Geometry check sheet. Reference: the model listing, model coordinates, mm. A direction names the side the tool comes from. Round coordinates to 2 decimals unless told otherwise and drop trailing zeros. Write each loop counter-clockwise with the first axis right and the second up, starting at its lowest first coordinate (ties: lowest second). Pieces come first, ordered by that corner, then holes. Notation, with made-up numbers: (46, -2.75) -> (70, -2.75) arc R11 ccw to (70, 2.25) -> close; hole circle Ø10 at (50.25, -6.75). An arc over 180 degrees is marked (long way). One line per question, with ' | ' between items.
```python
from build123d import *

# Parameters (mm, degrees)
SKETCH1_W                 = 50.8
SKETCH1_H                 = 126.238
BACK_DEPTH                = 3.175
CUT_EXTRUDE3_DEPTH        = 69.11203114
F_4_CLEARANCE_HOLE1_D     = 3.4544
LPATTERN1_OUTLINE_R       = 1.7272
LPATTERN1_DEPTH           = 3.175
SKETCH9_W                 = 55.88
SKETCH9_H                 = 131.318
WALLS_DEPTH               = 11.405821857
SKETCH11_W                = 69.85
SKETCH11_H                = 137.668
SKETCH11_W_2              = 50.8
SKETCH11_H_2              = 126.238
LIP_DEPTH                 = 2.54
F_6_CLEARANCE_OVERSIZED_D = 4.3053
FILLET2_R                 = 1.5875
CUT_EXTRUDE4_DEPTH        = 6.858
CUT_EXTRUDE4_DEPTH_BACK   = 3.81
SKETCH19_W                = 76.814856898
SKETCH19_H                = 21.095936882


# Read off the part's stored shape, not the designer's step: LPattern1
with BuildPart() as part:
    # Sketch1 → back (new body)
    with BuildSketch(Plane.XY):
        Rectangle(SKETCH1_W, SKETCH1_H)
    extrude(amount=BACK_DEPTH)

    # Sketch6 → Cut-Extrude3 (cut, through all)
    with BuildSketch(Plane.XY.offset(3.175)):
        with BuildLine():
            Line((24.07, -52.705), (24.07, 52.705))
            ThreePointArc((24.07, 52.705), (23.605032015, 53.827532015), (22.4825, 54.2925))
            Line((22.4825, 54.2925), (15.6245, 54.2925))
            ThreePointArc((15.6245, 54.2925), (14.501967985, 53.827532015), (14.037, 52.705))
            Line((14.037, 52.705), (14.037, -52.705))
            ThreePointArc((14.037, -52.705), (14.501967985, -53.827532015), (15.6245, -54.2925))
            Line((15.6245, -54.2925), (22.4825, -54.2925))
            ThreePointArc((22.4825, -54.2925), (23.605032015, -53.827532015), (24.07, -52.705))
        make_face()
    extrude(amount=-CUT_EXTRUDE3_DEPTH, mode=Mode.SUBTRACT)

    # #4 Clearance Hole1 (through all)
    with Locations(Plane(origin=(19.0535, 58.1025, 3.175), x_dir=(1, 0, 0), z_dir=(0, 0, 1))):
        with Locations((0, 0), (0, -116.205)):
            Hole(F_4_CLEARANCE_HOLE1_D / 2)

    # LPattern1 outline → LPattern1 (cut)
    with BuildSketch(Plane.XY):
        with BuildLine():
            ThreePointArc((1.337, -52.705), (1.801967985, -53.827532015), (2.9245, -54.2925))
            Line((2.9245, -54.2925), (9.7825, -54.2925))
            ThreePointArc((9.7825, -54.2925), (10.905032015, -53.827532015), (11.37, -52.705))
            Line((11.37, -52.705), (11.37, 52.705))
            ThreePointArc((11.37, 52.705), (10.905032015, 53.827532015), (9.7825, 54.2925))
            Line((9.7825, 54.2925), (2.9245, 54.2925))
            ThreePointArc((2.9245, 54.2925), (1.801967985, 53.827532015), (1.337, 52.705))
            Line((1.337, 52.705), (1.337, -52.705))
        make_face()
        with BuildLine():
            ThreePointArc((-11.363, -52.705), (-10.898032015, -53.827532015), (-9.7755, -54.2925))
            Line((-9.7755, -54.2925), (-2.9175, -54.2925))
            ThreePointArc((-2.9175, -54.2925), (-1.794967985, -53.827532015), (-1.33, -52.705))
            Line((-1.33, -52.705), (-1.33, 52.705))
            ThreePointArc((-1.33, 52.705), (-1.794967985, 53.827532015), (-2.9175, 54.2925))
            Line((-2.9175, 54.2925), (-9.7755, 54.2925))
            ThreePointArc((-9.7755, 54.2925), (-10.898032015, 53.827532015), (-11.363, 52.705))
            Line((-11.363, 52.705), (-11.363, -52.705))
        make_face()
        with BuildLine():
            ThreePointArc((-24.063, -52.705), (-23.598032015, -53.827532015), (-22.4755, -54.2925))
            Line((-22.4755, -54.2925), (-15.6175, -54.2925))
            ThreePointArc((-15.6175, -54.2925), (-14.494967985, -53.827532015), (-14.03, -52.705))
            Line((-14.03, -52.705), (-14.03, 52.705))
            ThreePointArc((-14.03, 52.705), (-14.494967985, 53.827532015), (-15.6175, 54.2925))
            Line((-15.6175, 54.2925), (-22.4755, 54.2925))
            ThreePointArc((-22.4755, 54.2925), (-23.598032015, 53.827532015), (-24.063, 52.705))
            Line((-24.063, 52.705), (-24.063, -52.705))
        make_face()
        with Locations((6.3535, -58.1025)):
            Circle(LPATTERN1_OUTLINE_R)
        with Locations((-6.3465, -58.1025)):
            Circle(LPATTERN1_OUTLINE_R)
        with Locations((-19.0465, -58.1025)):
            Circle(LPATTERN1_OUTLINE_R)
        with Locations((6.3535, 58.1025)):
            Circle(LPATTERN1_OUTLINE_R)
        with Locations((-6.3465, 58.1025)):
            Circle(LPATTERN1_OUTLINE_R)
        with Locations((-19.0465, 58.1025)):
            Circle(LPATTERN1_OUTLINE_R)
    extrude(amount=LPATTERN1_DEPTH, mode=Mode.SUBTRACT)

    # Sketch9 → walls (add)
    with BuildSketch(Plane.XY.offset(3.175)):
        Rectangle(SKETCH9_W, SKETCH9_H)
        with BuildLine():
            Line((25.4, -61.5315), (25.4, 61.5315))
            ThreePointArc((25.4, 61.5315), (24.935032015, 62.654032015), (23.8125, 63.119))
            Line((23.8125, 63.119), (-23.8125, 63.119))
            ThreePointArc((-23.8125, 63.119), (-24.935032015, 62.654032015), (-25.4, 61.5315))
            Line((-25.4, 61.5315), (-25.4, -61.5315))
            ThreePointArc((-25.4, -61.5315), (-24.935032015, -62.654032015), (-23.8125, -63.119))
            Line((-23.8125, -63.119), (23.8125, -63.119))
            ThreePointArc((23.8125, -63.119), (24.935032015, -62.654032015), (25.4, -61.5315))
        make_face(mode=Mode.SUBTRACT)
    extrude(amount=-WALLS_DEPTH)

    # Sketch11 → lip (add)
    with BuildSketch(Plane(origin=(0, 0, -8.230821857), x_dir=(-1, 0, 0), z_dir=(0, 0, -1))):
        Rectangle(SKETCH11_W, SKETCH11_H)
        Rectangle(SKETCH11_W_2, SKETCH11_H_2, mode=Mode.SUBTRACT)
    extrude(amount=-LIP_DEPTH)

    # #6 Clearance OVERSIZED (through all)
    with Locations(Plane(origin=(-31.4325, 44.45, -5.690821857), x_dir=(1, 0, 0), z_dir=(0, 0, 1))):
        with Locations((0, 0), (0, -44.45), (0, -88.9)):
            f_6_clearance_oversized = Hole(F_6_CLEARANCE_OVERSIZED_D / 2)

    # Fillet2
    fillet2_edges = [part.edges().sort_by_distance(p)[0] for p in [
        (34.925, 68.834, -6.960821857),
        (-34.925, 68.834, -6.960821857),
        (-34.925, -68.834, -6.960821857),
        (34.925, -68.834, -6.960821857),
    ]]
    fillet(fillet2_edges, radius=FILLET2_R)

    # Mirror2: #6 Clearance OVERSIZED across plane
    add(f_6_clearance_oversized.mirror(Plane(origin=(0, 0, 0), x_dir=(0, 0, 1), z_dir=(1, 0, 0))), mode=Mode.SUBTRACT)

    # Sketch19 → Cut-Extrude4 (cut, two sides: drawn at the far end of the back side and taken through both)
    with BuildSketch(Plane(origin=(0, 65.659, 0), x_dir=(1, 0, 0), z_dir=(0, 1, 0)).offset(-CUT_EXTRUDE4_DEPTH_BACK)):
        Rectangle(SKETCH19_W, SKETCH19_H)
    extrude(amount=CUT_EXTRUDE4_DEPTH + CUT_EXTRUDE4_DEPTH_BACK, mode=Mode.SUBTRACT)


solid = part.part
```
(1) Sectioned sample at B-B on y = 15. Record the cut outline in (x, z) (3 decimals).
Resolved:
outline: (-34.925, -8.231) -> (-25.4, -8.231) -> (-25.4, 0) -> (-24.063, 0) -> (-24.063, 3.175) -> (-27.94, 3.175) -> (-27.94, -5.691) -> (-34.925, -5.691) -> close; (-14.03, 0) -> (-11.363, 0) -> (-11.363, 3.175) -> (-14.03, 3.175) -> close; (-1.33, 0) -> (1.337, 0) -> (1.337, 3.175) -> (-1.33, 3.175) -> close; (11.37, 0) -> (14.037, 0) -> (14.037, 3.175) -> (11.37, 3.175) -> close; (24.07, 0) -> (25.4, 0) -> (25.4, -8.231) -> (34.925, -8.231) -> (34.925, -5.691) -> (27.94, -5.691) -> (27.94, 3.175) -> (24.07, 3.175) -> close
(2) Access from +Z, -Z, +X, -X, +Y, -Y to the whole of each face (thin tool, end or side, straight path). Record for faces 4 (the flat face through (-6, -54.292, 2)), 5 (the flat face through (0, -65.659, -1)), 6 (the flat face through (0, -68.834, -7)).
Resolved:
face 4: +Z, -Z | face 5: +Z, +X, -X, -Y | face 6: +Z, -Z, +X, -X, -Y
(3) Material ranges on line 1 (X direction, y = 12, z = -5); line 2 (Y direction, x = 15, z = -3.5); line 3 (X direction, y = -60, z = 0.75), recorded low to high.
Resolved:
line 1: x = -27.94 to -25.4, 25.4 to 27.94 | line 2: y = -65.66 to -63.12 | line 3: x = -27.94 to 27.94
(4) Sectioned sample at A-A on z = -7. Count the separate pieces of the cut face and the enclosed holes in it, then the cut area to 3 significant figures.
Resolved:
separate pieces: 1 | enclosed holes: 6 | area: 2,690 mm2
(5) Draft check along X on faces 1 (the flat face through (25.4, -1, -4)), 2 (the flat face through (34.925, -4, -7)), 3 (the flat face through (26, -13, -8.231)). Enter one of: +X half, -X half, draft (parallel to the pull), parting line (faces both ways), or undercut.
Resolved:
face 1: undercut | face 2: +X half | face 3: draft
(6) Go/stop test with flat-tipped pins: pin 1 (3.5 mm diameter, centred on y = -25.5, z = 2, fed in from -X); pin 2 (1.6 mm diameter, centred on y = -15, z = 2, fed in from +X); pin 3 (1.6 mm diameter, centred on x = 17.5, z = 1, fed in from -Y). Record where each tip stops, or that it passes through.
Resolved:
pin 1: stops at x = -27.94 | pin 2: stops at x = 27.94 | pin 3: stops at y = -65.66
